Model file for the job. Use its own axes, mm. Face numbers are marked on the shaded views. A direction names the side the tool comes from. Coordinates: 2 decimals unless noted, no trailing zeros. Loops run counter-clockwise (first coordinate to the right, second up) from the corner with the lowest first, then second, coordinate; pieces in that order, holes last.
Autodesk Inventor part; units mm, degrees
ref_plane "YZ Plane" through (0, 0, 0) normal (1, 0, 0) x (0, 1, 0)
ref_plane "XZ Plane" through (0, 0, 0) normal (0, 1, 0) x (-1, 0, 0)
ref_plane "XY Plane" through (0, 0, 0) normal (0, 0, 1) x (1, 0, 0)
sketch "Sketch1" plane through (0, 0, 0) normal (0, 1, 0) x (-1, 0, 0)
  line L0 (123.19, 31.75) -> (-123.19, 31.75)
  line L1 (-123.19, 31.75) -> (-123.19, -31.75)
  line L2 (-123.19, -31.75) -> (123.19, -31.75)
  line L3 (123.19, -31.75) -> (123.19, 31.75)
  line L4 (123.19, 31.75) -> (-123.19, -31.75) construction
  line L5 (-123.19, 31.75) -> (123.19, -31.75) construction
  point P0 (0, 0)
  dimension "d0" = 246.38
  dimension "d1" = 63.5
extrude "Extrusion1" add sketch "Sketch1" against normal blind 12.7
sketch "Sketch2" plane through (0, 0, 0) normal (0, 1, 0) x (1, 0, 0)
  line L0 (-123.19, -31.75) -> (-123.19, 31.75)
  line L1 (-123.19, 31.75) -> (123.19, 31.75)
  line L2 (-123.19, -31.75) -> (-110.49, -31.75)
  line L3 (-110.49, -31.75) -> (-110.49, 31.75)
  line L4 (-110.49, 31.75) -> (-123.19, 31.75)
  line L5 (-123.19, 31.75) -> (-123.19, -31.75)
  line L6 (123.19, 31.75) -> (123.19, -31.75)
  line L7 (123.19, -31.75) -> (110.49, -31.75)
  line L8 (110.49, -31.75) -> (110.49, 31.75)
  line L9 (110.49, 31.75) -> (123.19, 31.75)
  line L10 (123.19, 31.75) -> (123.19, -31.75)
  point P0 (0, 0)
  dimension "d4" = 12.7
  dimension "d5" = 12.7
extrude "Extrusion2" add sketch "Sketch2" along normal blind 215.9
sketch "Sketch3" plane through (-123.19, -12.7, -31.75) normal (-1, 0, 0) x (0, 0, 1)
  line L0 (0, 228.6) -> (63.5, 228.6) construction
  line L1 (31.75, 228.6) -> (31.75, 0) construction
  line L2 (63.5, 0) -> (0, 0) construction
  circle A0 centre (31.75, 209.55) radius 12.7
  line L3 (0, 12.7) -> (0, 228.6) construction
  line L4 (0, 222.25) -> (38.1, 222.25) construction
  point P0 (31.75, 12.7)
  dimension "d8" = 25.4
  dimension "d9" = 6.35
extrude "Extrusion3" cut sketch "Sketch3" against normal through all
sketch "Sketch4" plane through (0, 0, 0) normal (0, 1, 0) x (1, 0, 0)
  line L0 (6.35, 3.6662) -> (6.35, -3.6662)
  line L1 (6.35, -3.6662) -> (0, -7.3323)
  line L2 (0, -7.3323) -> (-6.35, -3.6662)
  line L3 (-6.35, -3.6662) -> (-6.35, 3.6662)
  line L4 (-6.35, 3.6662) -> (0, 7.3323)
  line L5 (0, 7.3323) -> (6.35, 3.6662)
  point P0 (0, 0)
  point P1 (0, 0)
  dimension "d13" = 12.7
extrude "Extrusion4" cut sketch "Sketch4" against normal through all
properties part number "forkV03" material "PBT Plastic"
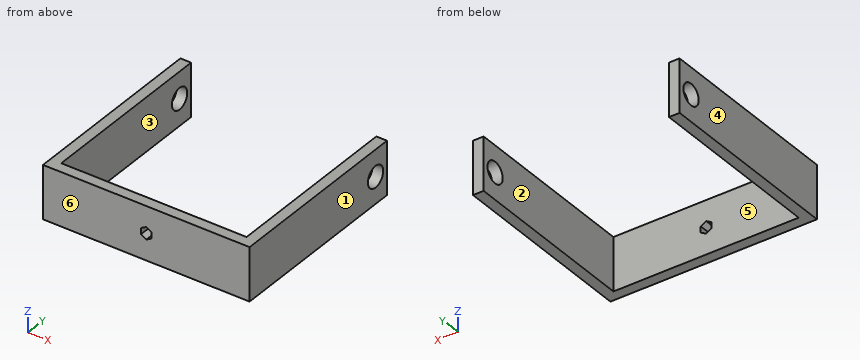
Q1. Slice it at C-C (y = 196.85). List the corners of the cut face in (x, z).
Answers:
outline: (-123.19, -31.75) - (-110.49, -31.75) - (-110.49, -12.7) - (-123.19, -12.7) - close; (-123.19, 12.7) - (-110.49, 12.7) - (-110.49, 31.75) - (-123.19, 31.75) - close; (110.49, -31.75) - (123.19, -31.75) - (123.19, -12.7) - (110.49, -12.7) - close; (110.49, 12.7) - (123.19, 12.7) - (123.19, 31.75) - (110.49, 31.75) - close
Q2. Slice it at A-A (z = 0). List the corners of the cut face in (x, y), and give its area (3 significant figures).
Answers:
outline: (-123.19, -12.7) - (-6.35, -12.7) - (-6.35, 0) - (-110.49, 0) - (-110.49, 184.15) - (-123.19, 184.15) - close; (-123.19, 209.55) - (-110.49, 209.55) - (-110.49, 215.9) - (-123.19, 215.9) - close; (6.35, -12.7) - (123.19, -12.7) - (123.19, 184.15) - (110.49, 184.15) - (110.49, 0) - (6.35, 0) - close; (110.49, 209.55) - (123.19, 209.55) - (123.19, 215.9) - (110.49, 215.9) - close
area: 7,810 mm2
Q3. Which spindle directions (+Z, -Z, +X, -X, +Y, -Y) get a long thin tool onto all of the face, cutting with end or side? Do the marked faces 5 and 6. Say none if no direction does.
Answers:
face 5: +Z, -Z, +Y
face 6: +Z, -Z, +X, -X, -Y
Q4. Flat gauge pin, fed straight in: P1, Ø8, axis at x = 83.5, z = 10.5, coming from the +Y side. Where does the tip first touch, or does it go through?
Answers:
P1: stops at y = 0
Q5. Slice it at D-D (z = 24.5). List the corners of the cut face in (x, y), and give its area (3 significant figures).
Answers:
outline: (-123.19, -12.7) - (123.19, -12.7) - (123.19, 215.9) - (110.49, 215.9) - (110.49, 0) - (-110.49, 0) - (-110.49, 215.9) - (-123.19, 215.9) - close
area: 8,610 mm2
Q6. Mould opens along X. For the marked faces 1, 2, 3 and 4 say: +X half, -X half, draft (parallel to the pull), parting line (faces both ways), or undercut.
Answers:
face 1: +X half
face 2: undercut
face 3: undercut
face 4: -X half
Q7. Drill centre lines: line 1 (X direction, y = 17.5, z = -7.5); line 2 (Y direction, x = -116, z = 0); line 3 (Z direction, x = 118, y = 196). Where is each one in solid material? Low to high.
Answers:
line 1: x = -123.19 to -110.49, 110.49 to 123.19
line 2: y = -12.7 to 184.15, 209.55 to 215.9
line 3: z = -31.75 to -12.67, 12.67 to 31.75
Q8. Slice it at B-B (y = 43). List the corners of the cut face in (x, z).
Answers:
outline: (-123.19, -31.75) - (-110.49, -31.75) - (-110.49, 31.75) - (-123.19, 31.75) - close; (110.49, -31.75) - (123.19, -31.75) - (123.19, 31.75) - (110.49, 31.75) - close
